from build123d import *

# Parameters (mm, degrees)
M7X1_0_1_D               = 6
M7X1_0_1_DEPTH           = 15
SKETCH_6_R               = 1
CUT_EXTRUDE_1_DEPTH      = 15
CUT_EXTRUDE_2_DEPTH      = 46.518512717
CUT_EXTRUDE_2_DEPTH_BACK = 46.518512717
SKETCH_8_R               = 4


with BuildPart() as part:
    # 草图1 → 旋转1 (revolve)
    with BuildSketch(Plane.XY, mode=Mode.PRIVATE) as revolve_1_sk:
        Polygon((0, 0), (11.15, 0), (11.15, 0.9), (7, 0.9), (7, 2.5), (11.15, 2.5), (11.15, 3.4), (6.5, 3.4), (6.5, 5), (11.15, 5), (11.15, 5.9), (6.3, 5.9), (6.3, 7.5), (11.15, 7.5), (11.15, 8.4), (6.1, 8.4), (6.1, 10), (11.15, 10), (11.15, 10.9), (5.9, 10.9), (5.9, 12.5), (11.15, 12.5), (11.15, 13.4), (5.7, 13.4), (5.7, 15), (11.15, 15), (11.15, 15.9), (5.5, 15.9), (5.5, 17.5), (11.15, 17.5), (11.15, 18.4), (5.3, 18.4), (5.3, 20), (11.15, 20), (11.15, 20.9), (5.1, 20.9), (5.1, 22.5), (11.15, 22.5), (11.15, 23.4), (4.9, 23.4), (4.9, 25), (11.15, 25), (11.15, 25.9), (4.7, 25.9), (4.7, 27.4), (8, 27.4), (8, 28.3), (4.5, 28.3), (4.5, 30.3), (8, 30.3), (8, 32.8), (6, 32.8), (6, 38.8), (8, 38.8), (8, 42.7), (0, 42.7), align=None)
    revolve(revolve_1_sk.sketch.rotate(Axis((0, 42.7, 0), (0, -1, 0)), 180), axis=Axis((0, 42.7, 0), (0, -1, 0)))

    # 草图2 → 1/8 Rc 螺纹孔1 (revolve, cut)
    with BuildSketch(Plane(origin=(0, 42.7, 0), x_dir=(0, 0, 1), z_dir=(1, 0, 0))):
        Polygon((0, 0), (0, 11.373399445), (3.95, 9), (3.95, 8), (4.342497031, 8), (4.59223, 0), align=None)
    revolve(axis=Axis((0, 49.05, 0), (0, -1, 0)), mode=Mode.SUBTRACT)

    # M7x1.0 螺纹孔1
    with Locations(Plane(origin=(0, 0, 0), x_dir=(-1, 0, 0), z_dir=(0, -1, 0))):
        with Locations((0, 0)):
            Hole(M7X1_0_1_D / 2, depth=M7X1_0_1_DEPTH)

    # 草图6 → 切除-拉伸1 (cut)
    with BuildSketch(Plane.XZ.offset(-15)):
        with Locations(Location((0, 0, 0), (0, 0, 270))):
            Circle(SKETCH_6_R)
    extrude(amount=-CUT_EXTRUDE_1_DEPTH, mode=Mode.SUBTRACT)

    # 草图8 → 切除-拉伸2 (cut, two sides: drawn at the far end of the back side and taken through both)
    with BuildSketch(Plane(origin=(0, 42.7, 0), x_dir=(1, 0, 0), z_dir=(0, 1, 0)).offset(-CUT_EXTRUDE_2_DEPTH_BACK)):
        with Locations(Location((0, 0, 0), (0, 0, 180))):
            Circle(SKETCH_8_R)
    extrude(amount=CUT_EXTRUDE_2_DEPTH + CUT_EXTRUDE_2_DEPTH_BACK, mode=Mode.SUBTRACT)


solid = part.part
CAD build for the part. Positions are in the model's coordinates, mm. A direction names the side the tool comes from. Give positions to 0.01 mm unless a question says otherwise; leave off trailing zeros. Write each loop counter-clockwise with the first axis right and the second up, starting at its lowest first coordinate (ties: lowest second). Pieces come first, ordered by that corner, then holes. Notation, with made-up numbers: (63, 47.5) - (97, 47.5) arc R26 ccw to (97, 74.5) - close; hole circle Ø6 at (-9, 24.5). An arc over 180 degrees is marked (long way). Answer as CSV lines item,"result".
Q1. Band-saw the part on A-A (y = 12). Give the cut face in (x, z).
Result set:
outline,"circle Ø11.8 at (0, 0); hole circle Ø8 at (0, 0)"
Q2. Band-saw the part on C-C (y = 4.5). Give the cut face in (x, z).
Result set:
outline,"circle Ø13 at (0, 0); hole circle Ø8 at (0, 0)"
Q3. 3-axis set-ups, long thin cutter, end or side, ignore diameter. For faces 1 (the face through (5, 5, 5)), 2 (the face through (0.867, 17.107, -3.905)): which of +Z, -Z, +X, -X, +Y, -Y reach the whole face in a straight line?
Result set:
face 1,"none"
face 2,"+Y, -Y"
Q4. Drill centre lines: line 1 (Y direction, x = -3.25, z = -4.25); line 2 (Z direction, x = 0, y = 27); line 3 (Z direction, x = 0, y = 27.5). Where is each one in solid material? Low to high. Write a range as from..to.
Result set:
line 1,"0..18.4, 20..20.9, 22.5..23.4, 25..25.9, 27.4..28.3, 30.3..42.7"
line 2,"-4.7..-4, 4..4.7"
line 3,"-8..-4, 4..8"
Q5. Flat gauge pins, fed straight in: pin 1 Ø13 at (x, z) = (-0.5, -1.5) entering from -Y; pin 2 Ø1.5 at (x, y) = (-3.5, 10) entering from +Z; pin 3 Ø8 at (y, z) = (29, 4.5) entering from -X; pin 4 Ø6 at (y, z) = (17, -5.5) entering from +X. Where does each tip first touch, or does it go through?
Result set:
pin 1,"y = 0"
pin 2,"z = 10.81"
pin 3,"x = -10.97"
pin 4,"x = 10.86"
Q6. Band-saw the part on B-B (z = 9.5). State how many separate pieces and enclosed holes the cut face has, and give its area (3 significant figures).
Result set:
separate pieces,"11"
enclosed holes,"0"
area,"116 mm²"
Q7. Pull direction Y, two halves, no side cores. Call faces 3 (the face through (1.73, 40.78, 7.81)), 4 (the face through (1.236, 14.211, 5.564)), 5 (the face through (4.363, 38.756, -0.969)): released by +Y, released by -Y, zero draft, split by the parting line, or undercut.
Result set:
face 3,"zero draft"
face 4,"undercut"
face 5,"released by +Y"
